```python
from build123d import *

# Parameters (mm, degrees)
SKETCH003_W  = 90
SKETCH003_H  = 13
PAD003_DEPTH = 2
SKETCH002_W  = 60
SKETCH002_H  = 13
PAD002_DEPTH = 2
SKETCH_W     = 90
SKETCH_H     = 60
SKETCH_R     = 2.5
SKETCH_W_2   = 18
SKETCH_H_2   = 18
SKETCH_W_3   = 15.3
SKETCH_H_3   = 20
PAD_DEPTH    = 2
SKETCH001_W  = 90
SKETCH001_H  = 13
PAD001_DEPTH = 2
SKETCH004_W  = 60
SKETCH004_H  = 13
PAD004_DEPTH = 2


with BuildPart() as body003:
    # Sketch003 → Pad003 (new body)
    with BuildSketch(Plane.XZ):
        with Locations((0, 6.5)):
            Rectangle(SKETCH003_W, SKETCH003_H)
    extrude(amount=PAD003_DEPTH)


with BuildPart() as body003_1:
    # Body003 placement: moved
    add(body003.part.moved(Location((0, -30, 0))))


with BuildPart() as body002:
    # Sketch002 → Pad002 (new body)
    with BuildSketch(Plane.YZ):
        with Locations((0, 6.5)):
            Rectangle(SKETCH002_W, SKETCH002_H)
    extrude(amount=PAD002_DEPTH)


with BuildPart() as body002_1:
    # Body002 placement: moved
    add(body002.part.moved(Location((43, 0, 0))))


with BuildPart() as body:
    # Sketch → Pad (new body)
    with BuildSketch(Plane.XY):
        Rectangle(SKETCH_W, SKETCH_H)
        with Locations((-40, 25)):
            Circle(SKETCH_R, mode=Mode.SUBTRACT)
        with Locations((-40, -25)):
            Circle(SKETCH_R, mode=Mode.SUBTRACT)
        with Locations((40, -25)):
            Circle(SKETCH_R, mode=Mode.SUBTRACT)
        with Locations((40, 25)):
            Circle(SKETCH_R, mode=Mode.SUBTRACT)
        with Locations((18, 15)):
            Circle(SKETCH_R, mode=Mode.SUBTRACT)
        with Locations((17, -9)):
            Rectangle(SKETCH_W_2, SKETCH_H_2, mode=Mode.SUBTRACT)
        with Locations((-22.35, 0)):
            Rectangle(SKETCH_W_3, SKETCH_H_3, mode=Mode.SUBTRACT)
    extrude(amount=PAD_DEPTH)


with BuildPart() as body001:
    # Sketch001 → Pad001 (new body)
    with BuildSketch(Plane.XZ):
        with Locations((0, 6.5)):
            Rectangle(SKETCH001_W, SKETCH001_H)
    extrude(amount=PAD001_DEPTH)


with BuildPart() as body001_1:
    # Body001 placement: moved
    add(body001.part.moved(Location((0, 30, 0))))


with BuildPart() as fusion001:
    # Fusion base: copy of Body
    add(body.part)

    # Fusion: union Body001
    add(body001_1.part)

    # Fusion001: union Body002, Body, Body001
    add(body002_1.part)
    add(body.part)
    add(body001_1.part)


with BuildPart() as fusion002:
    # Fusion002 base: copy of Fusion001
    add(fusion001.part)

    # Fusion002: union Body003
    add(body003_1.part)


with BuildPart() as body004:
    # Sketch004 → Pad004 (new body)
    with BuildSketch(Plane.YZ):
        with Locations((0, 6.5)):
            Rectangle(SKETCH004_W, SKETCH004_H)
    extrude(amount=PAD004_DEPTH)


with BuildPart() as body004_1:
    # Body004 placement: moved
    add(body004.part.moved(Location((-45, 0, 0))))


with BuildPart() as fusion004:
    # Fusion003 base: copy of Fusion002
    add(fusion002.part)

    # Fusion003: union Body004
    add(body004_1.part)

    # Fusion004: union Fusion002, Body004, Fusion001, Body003
    add(fusion002.part)
    add(body004_1.part)
    add(fusion001.part)
    add(body003_1.part)


solid = fusion004.part
```
Could you check a few things on this model? Use its own coordinates, in mm. A direction names the side the tool comes from. Round coordinates to 2 decimals unless told otherwise and drop trailing zeros. Loops run counter-clockwise (first coordinate to the right, second up) from the corner with the lowest first, then second, coordinate; pieces in that order, holes last. Notation, with made-up numbers: (25, 47) - (57, 47) arc R24 cw to (57, 85) - close; hole circle Ø10 at (35.5, 38.25). An arc over 180 degrees is marked (long way). Answer as CSV lines item,"result".
1. I want a section at D-D on z = 3. List the corners of the cut face in (x, y) for me, then the cut area to 3 significant figures.
Filled in:
outline,"(-45, -32) - (45, -32) - (45, 30) - (-45, 30) - close; hole (-43, -30) - (43, -30) - (43, 28) - (-43, 28) - close"
area,"592 mm^2"
2. I want a section at A-A on x = 18. List the corners of the cut face in (y, z) for me.
Filled in:
outline,"(-32, 0) - (-18, 0) - (-18, 2) - (-30, 2) - (-30, 13) - (-32, 13) - close; (0, 0) - (12.5, 0) - (12.5, 2) - (0, 2) - close; (17.5, 0) - (30, 0) - (30, 13) - (28, 13) - (28, 2) - (17.5, 2) - close"
3. We'd pull the mould along X, two halves only. Please class faces 4 (the face through (45, -1, 6)), 5 (the face through (-4, -31, 13)), 6 (the face through (-22, 10, 1)): +X half, -X half, draft (parallel to the pull), parting line (faces both ways), or undercut.
Filled in:
face 4,"+X half"
face 5,"draft"
face 6,"undercut"
4. I want a section at C-C on x = -17. List the corners of the cut face in (y, z) for me, then the cut area to 3 significant figures.
Filled in:
outline,"(-32, 0) - (-10, 0) - (-10, 2) - (-30, 2) - (-30, 13) - (-32, 13) - close; (10, 0) - (30, 0) - (30, 13) - (28, 13) - (28, 2) - (10, 2) - close"
area,"128 mm^2"
5. Please list where these lines run through material, in increasing order: line 1 along Y through (x, z) = (18, 1.2); line 2 along Y through (x, z) = (-40, 0.9); line 3 along Y through (x, z) = (9, 4). Write a range as [from, to].
Filled in:
line 1,"y = [-32, -18], [0, 12.5], [17.5, 30]"
line 2,"y = [-32, -27.5], [-22.5, 22.5], [27.5, 30]"
line 3,"y = [-32, -30], [28, 30]"
6. For pin 1 Ø3 at (x, y) = (-22, -8) entering from +Z; pin 2 Ø1 at (x, y) = (-35.5, 8.5) entering from +Z, each with a flat end and sliding along its axis, tell me the tip position at first contact or that it passes through.
Filled in:
pin 1,"passes through"
pin 2,"stops at z = 2"
7. I want a section at B-B on y = -25. List the corners of the cut face in (x, z) for me.
Filled in:
outline,"(-45, 0) - (-42.5, 0) - (-42.5, 2) - (-43, 2) - (-43, 13) - (-45, 13) - close; (-37.5, 0) - (37.5, 0) - (37.5, 2) - (-37.5, 2) - close; (42.5, 0) - (45, 0) - (45, 13) - (43, 13) - (43, 2) - (42.5, 2) - close"
8. On a 3-axis mill with a long thin cutter (end or side, diameter ignored), from which of +Z, -Z, +X, -X, +Y, -Y can I reach the whole of each face in a straight line? I mean faces 1 (the face through (-1, -30, 8)), 2 (the face through (-1, 30, 6)), 3 (the face through (-30, 0, 1)). Say none if no direction works.
Filled in:
face 1,"+Z"
face 2,"+Z, -Z, +X, -X, +Y"
face 3,"+Z, -Z"
